Geometry check sheet. Reference: the model listing, model coordinates, mm. A direction names the side the tool comes from. Round coordinates to 2 decimals unless told otherwise and drop trailing zeros. Write each loop counter-clockwise with the first axis right and the second up, starting at its lowest first coordinate (ties: lowest second). Pieces come first, ordered by that corner, then holes. Notation, with made-up numbers: (0, 65.5) -> (28, 65.5) arc R13 cw to (28, 75.5) -> close; hole circle Ø3 at (13.25, 32). An arc over 180 degrees is marked (long way). Use a Markdown table: item, result.
```python
from build123d import *

# Parameters (mm, degrees)
BOSS_EXTRUDE1_DEPTH     = 6.35
CUT_EXTRUDE2_DEPTH      = 7.35
FILLET2_R               = 6.35
SKETCH4_W               = 6.35
SKETCH4_H               = 12.7
SKETCH4_H_2             = 4.7625
BOSS_EXTRUDE2_DEPTH     = 6.35
SKETCH5_W               = 13.97
SKETCH5_H               = 9.525
CUT_EXTRUDE3_DEPTH      = 7.35
FILLET3_R               = 3.175
F_1_4_CLEARANCE_HOLE1_D = 6.7564
BOSS_EXTRUDE3_DEPTH     = 6.35


with BuildPart() as part:
    # Sketch1 → Boss-Extrude1 (new body)
    with BuildSketch(Plane.XY):
        Polygon((-82.55, -19.05), (0, 0), (-88.9, 0), (-88.9, -19.05), align=None)
        Polygon((-95.25, 0), (0, 57.118902343), (0, 0), align=None)
    extrude(amount=BOSS_EXTRUDE1_DEPTH)

    # Sketch3 → Cut-Extrude2 (cut, through all)
    with BuildSketch(Plane.XY.offset(6.35)):
        Polygon((-82.55, -19.05), (-69.85, -3.175), (0, 25.4), (0, 0), align=None)
    extrude(amount=-CUT_EXTRUDE2_DEPTH, mode=Mode.SUBTRACT)

    # Fillet2
    fillet2_edges = [part.edges().sort_by_distance(p)[0] for p in [
        (-69.85, -3.175, 3.175),
    ]]
    fillet(fillet2_edges, radius=FILLET2_R)

    # Sketch4 → Boss-Extrude2 (add)
    with BuildSketch(Plane.XY.offset(6.35)):
        with Locations((3.175, 31.75)):
            Rectangle(SKETCH4_W, SKETCH4_H)
        with Locations((-92.075, -2.38125)):
            Rectangle(SKETCH4_W, SKETCH4_H_2)
    extrude(amount=-BOSS_EXTRUDE2_DEPTH)

    # Sketch5 → Cut-Extrude3 (cut, through all)
    with BuildSketch(Plane.XY.offset(6.35)):
        with Locations((-81.915, -14.2875)):
            Rectangle(SKETCH5_W, SKETCH5_H)
    extrude(amount=-CUT_EXTRUDE3_DEPTH, mode=Mode.SUBTRACT)

    # Fillet3
    fillet3_edges = [part.edges().sort_by_distance(p)[0] for p in [
        (-74.93, -9.525, 3.175),
    ]]
    fillet(fillet3_edges, radius=FILLET3_R)

    # 1/4 Clearance Hole1 (through all)
    with Locations(Plane.XY.offset(6.35)):
        with Locations((-79.884098694, 1.810281574), (-63.546505707, 11.607503394), (-47.20891272, 21.404725214)):
            Hole(F_1_4_CLEARANCE_HOLE1_D / 2)

    # Sketch8 → Boss-Extrude3 (add)
    with BuildSketch(Plane.XY.offset(6.35)):
        Polygon((-32.675185974, 37.524458703), (-34.308056278, 40.247390867), (-64.207684329, 22.317375804), (-62.574814026, 19.59444364), align=None)
    extrude(amount=-BOSS_EXTRUDE3_DEPTH)


solid = part.part
```
(1) Section check B-B on z = 3. State how many separate pieces and enclosed holes the cut face has, plus the area to 3 significant figures.
A:
| item | result |
|---|---|
| separate pieces | 1 |
| enclosed holes | 3 |
| area | 2,220 mm2 |
(2) Section check D-D on x = -10. Record the cut outline in (y, z), plus the area to 3 significant figures.
A:
| item | result |
|---|---|
| outline | (21.31, 0) -> (51.12, 0) -> (51.12, 6.35) -> (21.31, 6.35) -> close |
| area | 189 mm2 |
(3) Section check C-C on y = 36.5. Record the cut outline in (x, z).
A:
| item | result |
|---|---|
| outline | (-40.56, 0) -> (6.35, 0) -> (6.35, 6.35) -> (-40.56, 6.35) -> close |
(4) Access from +Z, -Z, +X, -X, +Y, -Y to the whole of each face (thin tool, end or side, straight path). Record for faces 5 (the face through (3, 25.4, 3)), 6 (the face through (-92, -4.762, 3)), 7 (the face through (-33.5, 38.9, 3.2)), 8 (the face through (6.35, 32, 3)), 9 (the face through (3, 38.1, 3)).
A:
| item | result |
|---|---|
| face 5 | +Z, -Z, +X, -Y |
| face 6 | +Z, -Z, -X, -Y |
| face 7 | +Z, -Z, +Y |
| face 8 | +Z, -Z, +X, +Y, -Y |
| face 9 | +Z, -Z, +X, +Y |
(5) Gauge pin test, flat ends, axial feed: pin 1 Ø1 at (x, z) = (-46.5, 3) entering from -Y; pin 2 Ø3 at (x, z) = (4.5, 2.5) entering from +Y; pin 3 Ø3 at (x, z) = (3.5, 4.5) entering from -Y. Record the tip position at first contact, or that the pin passes through.
A:
| item | result |
|---|---|
| pin 1 | stops at y = 6.17 |
| pin 2 | stops at y = 38.1 |
| pin 3 | stops at y = 25.4 |
(6) Release check for a two-part mould opening along X. For faces 1 (the face through (-60.17, 11.76, 3.13)), 2 (the face through (-46.5, 18.1, 3.1)), 3 (the face through (0, 48, 3)), 4 (the face through (-83, -9.525, 3)) record: +X half, -X half, draft (parallel to the pull), parting line (faces both ways), or undercut.
A:
| item | result |
|---|---|
| face 1 | undercut |
| face 2 | undercut |
| face 3 | +X half |
| face 4 | draft |
(7) Section check A-A on x = -79. Record the cut outline in (y, z) (3 decimals), plus the area to 3 significant figures.
A:
| item | result |
|---|---|
| outline | (-9.525, 0) -> (-1.45, 0) -> (-1.45, 6.35) -> (-9.525, 6.35) -> close; (5.071, 0) -> (9.745, 0) -> (9.745, 6.35) -> (5.071, 6.35) -> close |
| area | 81.0 mm2 |
(8) Thickness scan on line 1 (Y direction, x = -64, z = 4.5); line 2 (X direction, y = -0.5, z = 1); line 3 (X direction, y = 11.5, z = 5). Record the ranges inside material, lowest first.
A:
| item | result |
|---|---|
| line 1 | y = -0.78 to 8.26, 14.96 to 18.74, 21.97 to 22.44 |
| line 2 | x = -95.25 to -82.35, -77.42 to -63.31 |
| line 3 | x = -76.07 to -66.92, -60.17 to -33.98 |
